Here's how the part is built. I have some questions about the finished solid (model axes, mm). A direction names the side the tool comes from. Give positions to 0.01 mm unless a question says otherwise; leave off trailing zeros. Loops run counter-clockwise (first coordinate to the right, second up) from the corner with the lowest first, then second, coordinate; pieces in that order, holes last.
Q1. I need wall thicknesses on probe 1 along Z at (x, y) = (-40.5, 18.5); probe 2 along Y at (x, z) = (35, -5.5); probe 3 along X at (y, z) = (4, -44). Which ranges of each line are inside material? Lowest first, please.
Q2. Suppose I cut it at A-A (z = -54). List the corners of the cut face in (x, y) for me, and give its area (3 significant figures).
Q3. I'm going to push flat-ended pins straight in: P1, Ø1.9, axis at x = 61, y = 1.5, coming from the +Z side; P2, Ø7, axis at x = 66, y = 2, coming from the +Z side; P3, Ø7, axis at y = 2.5, z = 10, coming from the +X side; P4, Ø5, axis at y = 9, z = -45.5, coming from the -X side. Where does each tip first touch, or does it pass through?
Q4. Suppose I cut it at C-C (x = -60). List the corners of the cut face in (y, z) for me, and give its area (3 significant figures).
Q5. Thinking about a two-plate mould opening in Z: for faces 1 (the face through (57.15, 17, -64)), 2 (the face through (-7, 25, -63.5)), 3 (the face through (-60, 3, -57.15)), 4 (the face through (67, 3, 57.15)), which applies, pulls with the +Z half, pulls with the -Z half, needs draft (parallel to the pull), parting line crosses it, or undercut?
Q6. Suppose I cut it at B-B (y = 27). List the corners of the cut face in (x, z) for me, and give its area (3 significant figures).
Q7. For faces 5 (the face through (-60, 3, -31.75)), 6 (the face through (-67, 32.45, 67)), 7 (the face through (-67, 3, 38.1)), which set-ups out of +Z, -Z, +X, -X, +Y, -Y let a thin tool reach every point of the face, with its end or its side?
Q8. Suppose I cut it at D-D (y = 41). List the corners of the cut face in (x, z) for me (3 decimals), and give its area (3 significant figures).
```python
from build123d import *

# Parameters (mm, degrees)
SKETCH1_W                                  = 127
SKETCH1_H                                  = 139.7
BOSS_EXTRUDE1_DEPTH                        = 6.35
SKETCH3_W                                  = 127
SKETCH3_H                                  = 6.35
BOSS_EXTRUDE2_DEPTH                        = 38.1
BOSS_EXTRUDE3_DEPTH                        = 6.35
CUT_EXTRUDE2_DEPTH                         = 106.875658203
SKETCH8_R                                  = 1.65
CUT_EXTRUDE3_DEPTH                         = 12
MIRROR2_AT_THE_SECOND_PLANE_COPY_1_SKETC_R = 1.65
MIRROR2_AT_THE_SECOND_PLANE_COPY_1_DEPTH   = 12


with BuildPart() as part:
    # Sketch1 → Boss-Extrude1 (new body)
    with BuildSketch(Plane(origin=(0, 0, 0), x_dir=(1, 0, 0), z_dir=(0, 1, 0))):
        with Locations((-6.35, 0)):
            Rectangle(SKETCH1_W, SKETCH1_H)
    extrude(amount=BOSS_EXTRUDE1_DEPTH)

    # Sketch3 → Boss-Extrude2 (add)
    with BuildSketch(Plane(origin=(0, 6.35, 0), x_dir=(1, 0, 0), z_dir=(0, 1, 0))):
        with Locations((-6.35, 66.675)):
            Rectangle(SKETCH3_W, SKETCH3_H)
        with Locations((-6.35, -66.675)):
            Rectangle(SKETCH3_W, SKETCH3_H)
    extrude(amount=BOSS_EXTRUDE2_DEPTH)

    # Sketch6 → Boss-Extrude3 (add)
    with BuildSketch(Plane(origin=(0, 6.35, 0), x_dir=(1, 0, 0), z_dir=(0, 1, 0))):
        Polygon((57.15, 50.8), (63.5, 50.8), (63.5, 57.15), (69.85, 57.15), (69.85, 31.75), (63.5, 31.75), (63.5, 38.1), (57.15, 38.1), align=None)
    boss_extrude3 = extrude(amount=-BOSS_EXTRUDE3_DEPTH)

    # Sketch7 → Cut-Extrude2 (cut, through all)
    with BuildSketch(Plane(origin=(0, 6.35, 0), x_dir=(1, 0, 0), z_dir=(0, 1, 0))):
        Polygon((-69.85, 50.8), (-63.5, 50.8), (-63.5, 57.15), (-57.15, 57.15), (-57.15, 31.75), (-63.5, 31.75), (-63.5, 38.1), (-69.85, 38.1), align=None)
    cut_extrude2 = extrude(amount=-CUT_EXTRUDE2_DEPTH, mode=Mode.SUBTRACT)

    # Mirror1: Boss-Extrude3, Cut-Extrude2 across plane
    add(boss_extrude3.mirror(Plane.XY))
    add(cut_extrude2.mirror(Plane.XY), mode=Mode.SUBTRACT)

    # Sketch8 → Cut-Extrude3 (cut)
    with BuildSketch(Plane(origin=(0, 44.45, 0), x_dir=(1, 0, 0), z_dir=(0, 1, 0))):
        with Locations(Location((-66.675, 66.675, 0), (0, 0, 270))):
            Circle(SKETCH8_R)
    cut_extrude3 = extrude(amount=-CUT_EXTRUDE3_DEPTH, mode=Mode.SUBTRACT)

    # Mirror2: Cut-Extrude3 across plane
    add(cut_extrude3.mirror(Plane.XY), mode=Mode.SUBTRACT)

    # Mirror2 at the second plane: Cut-Extrude3 across plane
    add(cut_extrude3.mirror(Plane.ZY.offset(6.35)), mode=Mode.SUBTRACT)

    # Mirror2 at the second plane copy 1 sketc → Mirror2 at the second plane copy 1 (cut)
    with BuildSketch(Plane(origin=(-12.7, 44.45, 0), x_dir=(-1, 0, 0), z_dir=(0, 1, 0))):
        with Locations(Location((-66.675, 66.675, 0), (0, 0, 270))):
            Circle(MIRROR2_AT_THE_SECOND_PLANE_COPY_1_SKETC_R)
    extrude(amount=-MIRROR2_AT_THE_SECOND_PLANE_COPY_1_DEPTH, mode=Mode.SUBTRACT)


solid = part.part
```
Solutions:
1. probe 1: z = -69.85 to -63.5, 63.5 to 69.85
1. probe 2: y = 0 to 6.35
1. probe 3: x = -57.15 to 69.85
2. outline: (-69.85, 0) - (-63.5, 0) - (-63.5, 6.35) - (-69.85, 6.35) - close; (-57.15, 0) - (57.15, 0) - (57.15, 6.35) - (-57.15, 6.35) - close; (63.5, 0) - (69.85, 0) - (69.85, 6.35) - (63.5, 6.35) - close
2. area: 806 mm2
3. P1: stops at z = 50.8
3. P2: stops at z = 57.15
3. P3: stops at x = 57.15
3. P4: passes through
4. outline: (0, -69.85) - (44.45, -69.85) - (44.45, -63.5) - (6.35, -63.5) - (6.35, -57.15) - (0, -57.15) - close; (0, -31.75) - (6.35, -31.75) - (6.35, 31.75) - (0, 31.75) - close; (0, 57.15) - (6.35, 57.15) - (6.35, 63.5) - (44.45, 63.5) - (44.45, 69.85) - (0, 69.85) - close
4. area: 1,050 mm2
5. face 1: needs draft
5. face 2: undercut
5. face 3: undercut
5. face 4: pulls with the +Z half
6. outline: (-69.85, -69.85) - (57.15, -69.85) - (57.15, -63.5) - (-69.85, -63.5) - close; (-69.85, 63.5) - (57.15, 63.5) - (57.15, 69.85) - (-69.85, 69.85) - close
6. area: 1,610 mm2
7. face 5: +Y, -Y
7. face 6: +Y
7. face 7: -X, +Y, -Y
8. outline: (-69.85, -69.85) - (57.15, -69.85) - (57.15, -63.5) - (-69.85, -63.5) - close; (-69.85, 63.5) - (57.15, 63.5) - (57.15, 69.85) - (-69.85, 69.85) - close; hole circle Ø3.3 at (-66.675, -66.675); hole circle Ø3.3 at (-66.675, 66.675); hole circle Ø3.3 at (53.975, -66.675); hole circle Ø3.3 at (53.975, 66.675)
8. area: 1,580 mm2
